Autodesk Inventor part; units mm, degrees
ref_plane "YZ Plane" through (0, 0, 0) normal (1, 0, 0) x (0, 1, 0)
ref_plane "XZ Plane" through (0, 0, 0) normal (0, 1, 0) x (-1, 0, 0)
ref_plane "XY Plane" through (0, 0, 0) normal (0, 0, 1) x (1, 0, 0)
sketch "main" plane through (0, 0, 0) normal (0, 0, 1) x (1, 0, 0)
  circle A0 centre (5.5393, 31.9986) radius 2.1844
  circle A1 centre (5.5393, -31.5014) radius 2.1844
  arc A2 (11.8893, 31.9986) -> (-0.6874, 33.244) centre (5.5393, 31.9986) ccw
  arc A3 (-0.6874, -32.7467) -> (11.8893, -31.5014) centre (5.5393, -31.5014) ccw
  line L0 (11.8893, 31.9986) -> (11.8893, -31.5014)
  circle A4 centre (-0.8107, 0.2486) radius 2.1844
  arc A5 (-7.0374, 1.494) -> (-7.0374, -0.9967) centre (-0.8107, 0.2486) ccw
  line L1 (-0.6874, 33.244) -> (-7.0374, 1.494)
  line L2 (-7.0374, -0.9967) -> (-0.6874, -32.7467)
  point P0 (2.0663, 0.2486)
sketch "Sketch1" plane through (0, 0, 0) normal (0, 0, 1) x (1, 0, 0)
  circle A0 centre (0, 0) radius 2.1844
  circle A1 centre (63.5, -0.0173) radius 2.1844
  arc A2 (0.0017, 6.35) -> (-1.247, -6.2263) centre (0, 0) ccw
  arc A3 (64.7436, -6.2443) -> (63.5017, 6.3327) centre (63.5, -0.0173) ccw
  line L0 (0.0017, 6.35) -> (63.5017, 6.3327)
  circle A4 centre (31.7483, -6.3586) radius 2.1844
  arc A5 (30.5012, -12.585) -> (32.9919, -12.5857) centre (31.7483, -6.3586) ccw
  line L1 (-1.247, -6.2263) -> (30.5012, -12.585)
  line L2 (32.9919, -12.5857) -> (64.7436, -6.2443)
  point P0 (0, 0)
extrude "Extrusion1" add sketch "Sketch1" along normal blind 1.5875
properties part number "gearbox_gusset" material "Acetal Resin, White"
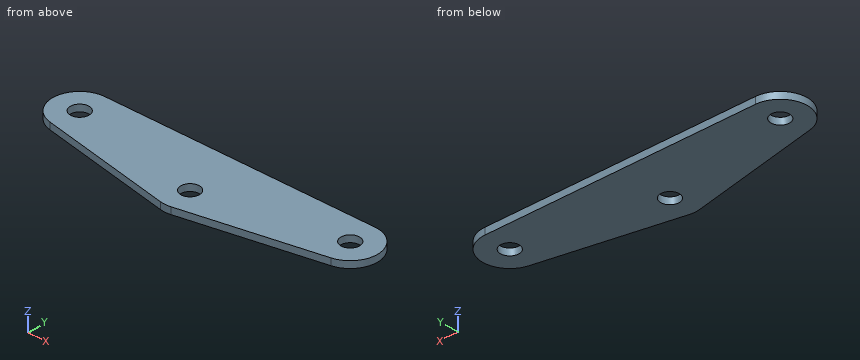
Work out the finished part from the listing and answer in its coordinate system (mm). Give positions to 0.01 mm unless a question says otherwise; leave off trailing zeros. Loops run counter-clockwise (first coordinate to the right, second up) from the corner with the lowest first, then second, coordinate; pieces in that order, holes last. Notation, with made-up numbers: (-26, -3) -> (-9, -3) arc R36 cw to (-9, 35) -> close; hole circle Ø7 at (34.5, 45.25). An arc over 180 degrees is marked (long way). Use a Markdown table: item, result. Add a question column.
1. Section A-A on z = 0.3 is taken. Determine the outline of the cut face in (x, y) (3 decimals).
2. Section C-C on x = 13 is taken. Determine the outline of the cut face in (y, z).
3. Flat-ended cylindrical pins translate along their axes: pin 1 Ø2.5 at (x, y) = (63.5, -0.02) entering from +Z; pin 2 Ø0.8 at (x, z) = (39.5, 0.5) entering from +Y. Find the tip coordinate at first contact, or state that the pin passes through.
4. Section B-B on y = 5.25 is taken. Determine the outline of the cut face in (x, z).
5. Find the intervals of material crossed by probe 1 along X at (y, z) = (0.25, 0.35); probe 2 along X at (y, z) = (1, 1.2); probe 3 along Y at (x, z) = (32, 1.1), in increasing order.
Results below:
| question | item | result |
|---|---|---|
| 1 | outline | (-1.247, -6.226) -> (30.501, -12.585) arc R6.35 ccw to (32.992, -12.586) -> (64.744, -6.244) arc R6.35 ccw to (63.502, 6.333) -> (0.002, 6.35) arc R6.35 ccw to start; hole circle Ø4.369 at (0, 0); hole circle Ø4.369 at (31.748, -6.359); hole circle Ø4.369 at (63.5, -0.017) |
| 2 | outline | (-9.08, 0) -> (6.35, 0) -> (6.35, 1.59) -> (-9.08, 1.59) -> close |
| 3 | pin 1 | passes through |
| 3 | pin 2 | stops at y = 6.34 |
| 4 | outline | (-3.57, 0) -> (67.05, 0) -> (67.05, 1.59) -> (-3.57, 1.59) -> close |
| 5 | probe 1 | x = -6.35 to -2.17, 2.17 to 61.33, 65.67 to 69.84 |
| 5 | probe 2 | x = -6.27 to -1.94, 1.94 to 61.57, 65.43 to 69.77 |
| 5 | probe 3 | y = -12.7 to -8.53, -4.19 to 6.34 |
